Geometry: final body of the model. Coordinates: model frame, mm. A direction names the side the tool comes from. Give positions to 0.01 mm unless a question says otherwise; leave off trailing zeros. Loops run counter-clockwise (first coordinate to the right, second up) from the corner with the lowest first, then second, coordinate; pieces in that order, holes last. Notation, with made-up numbers: (-4.75, -17.75) -> (50.25, -17.75) arc R14 cw to (50.25, -5.75) -> close; hole circle Ø3 at (-36, 13.25). An arc over 180 degrees is marked (long way). Answer in a Markdown table with one row per item. Add a question column.
1) Section query C-C (y = 87). Return the cut outline in (x, z), plus the area to 3 significant figures.
2) Section query B-B (x = 68.5). Return the cut outline in (y, z), plus the area to 4 significant figures.
3) Draft query along X for faces 1 (the flat face through (3, 0, 552)), 2 (the flat face through (254, 89, 552)), 3 (the flat face through (251, 92, 552)), 4 (the flat face through (-254, 91, 552)). Return one class per face: +X half, -X half, draft (parallel to the pull), parting line (faces both ways), or undercut.
4) First-contact query: P1, Ø12, axis at x = 115.5, z = 325, coming from the +Y side; P2, Ø2, axis at x = -30, z = 907, coming from the +Y side; P3, Ø1.5, axis at y = -1.5, z = 1005, coming from the -X side; P4, Ø0.9, axis at y = -1.5, z = 976, coming from the +X side. Flat tips, straight axial feed; report the tip coordinate or a pass-through.
5) Section query D-D (x = 0). Return the cut outline in (y, z), plus the area to 4 significant figures.
6) Access query for faces 5 (the cylindrical face through (-7.49, -1.52, 282.01)), 6 (the flat face through (-251, 90, 552)). Directions: +Z, -Z, +X, -X, +Y, -Y. A direction counts if a zero-diameter tool reaches every point of the face in a straight line with its end or side. Return the directions, or none.
7) Section query A-A (z = 360.5). Return the cut outline in (x, y), plus the area to 3 significant figures.
8) Line query: line 1 (X direction, y = -1.1, z = 325); line 2 (Z direction, x = 0, y = -2.15); line 3 (X direction, y = 53.5, z = 461). Output: solid intervals per line, ascending. Write a range as from..to.
```python
from build123d import *

# Parameters (mm, degrees)
F1_DEPTH = 1120
F2_R     = 57.5
F3_DEPTH = 183.001
F4_R     = 32.5
F5_DEPTH = 183.001
F7_DEPTH = 183.001
F8_R     = 7.5
F9_DEPTH = 183.001


with BuildPart() as f1:
    # F0 (on Top) → F1 (new body)
    with BuildSketch(Plane.XY):
        with BuildLine():
            Line((249, 0), (0, 0))
            Line((0, 0), (-249, 0))
            ThreePointArc((-249, 0), (-250.414214, 0.585786), (-251, 2))
            Line((-251, 2), (-251, 180))
            Line((-251, 180), (-254, 180))
            Line((-254, 180), (-254, 0))
            ThreePointArc((-254, 0), (-253.12132, -2.12132), (-251, -3))
            Line((-251, -3), (0, -3))
            Line((0, -3), (251, -3))
            ThreePointArc((251, -3), (253.12132, -2.12132), (254, 0))
            Line((254, 0), (254, 180))
            Line((254, 180), (251, 180))
            Line((251, 180), (251, 2))
            ThreePointArc((251, 2), (250.414214, 0.585786), (249, 0))
        make_face()
    extrude(amount=F1_DEPTH)

    # F2 (on face) → F3 (cut, through all)
    with BuildSketch(Plane.XZ.offset(3)):
        with Locations((0, 225)):
            Circle(F2_R)
    extrude(amount=-F3_DEPTH, mode=Mode.SUBTRACT)

    # F4 (on face) → F5 (cut, through all)
    with BuildSketch(Plane.XZ.offset(3)):
        with Locations((0, 360.5)):
            Circle(F4_R)
    extrude(amount=-F5_DEPTH, mode=Mode.SUBTRACT)

    # F6 (on face) → F7 (cut, through all)
    with BuildSketch(Plane.XZ.offset(3)):
        Polygon((-110, 927.5), (0, 927.5), (110, 927.5), (110, 1062.5), (0, 1062.5), (-110, 1062.5), align=None)
    extrude(amount=-F7_DEPTH, mode=Mode.SUBTRACT)

    # F8 (on face) → F9 (cut, through all)
    with BuildSketch(Plane.XZ.offset(3)):
        with Locations((-115.5, 325)):
            Circle(F8_R)
        with Locations((-89.5, 325)):
            Circle(F8_R)
        with Locations((89.5, 325)):
            Circle(F8_R)
        with Locations((115.5, 325)):
            Circle(F8_R)
    extrude(amount=-F9_DEPTH, mode=Mode.SUBTRACT)


solid = f1.part
```
Evaluation:
| question | item | result |
|---|---|---|
| 1 | outline | (-254, 0) -> (-251, 0) -> (-251, 1120) -> (-254, 1120) -> close; (251, 0) -> (254, 0) -> (254, 1120) -> (251, 1120) -> close |
| 1 | area | 6,720 mm² |
| 2 | outline | (-3, 0) -> (0, 0) -> (0, 927.5) -> (-3, 927.5) -> close; (-3, 1062.5) -> (0, 1062.5) -> (0, 1120) -> (-3, 1120) -> close |
| 2 | area | 2,955 mm² |
| 3 | face 1 | undercut |
| 3 | face 2 | +X half |
| 3 | face 3 | undercut |
| 3 | face 4 | -X half |
| 4 | P1 | through |
| 4 | P2 | y = 0 |
| 4 | P3 | x = -253.9 |
| 4 | P4 | x = 253.81 |
| 5 | outline | (-3, 0) -> (0, 0) -> (0, 167.5) -> (-3, 167.5) -> close; (-3, 282.5) -> (0, 282.5) -> (0, 328) -> (-3, 328) -> close; (-3, 393) -> (0, 393) -> (0, 927.5) -> (-3, 927.5) -> close; (-3, 1062.5) -> (0, 1062.5) -> (0, 1120) -> (-3, 1120) -> close |
| 5 | area | 2,415 mm² |
| 6 | face 5 | +Y, -Y |
| 6 | face 6 | +Z, -Z, +Y |
| 7 | outline | (-254, 0) arc R3 ccw to (-251, -3) -> (-32.5, -3) -> (-32.5, 0) -> (-249, 0) arc R2 cw to (-251, 2) -> (-251, 180) -> (-254, 180) -> close; (32.5, -3) -> (251, -3) arc R3 ccw to (254, 0) -> (254, 180) -> (251, 180) -> (251, 2) arc R2 cw to (249, 0) -> (32.5, 0) -> close |
| 7 | area | 2,410 mm² |
| 8 | line 1 | -253.79..-123, -108..-97, -82..82, 97..108, 123..253.79 |
| 8 | line 2 | 0..167.5, 282.5..328, 393..927.5, 1062.5..1120 |
| 8 | line 3 | -254..-251, 251..254 |
